Input: part model. Units: mm. Frame: model coordinates. A direction names the side the tool comes from. Round coordinates to 2 decimals unless told otherwise and drop trailing zeros. Order: outer loops, then holes, each group sorted by start corner. A loop starts at its lowest first (then second) coordinate and runs counter-clockwise, first axis right, second up. Notation, with made-up numbers: (25.5, -10) -> (84.5, -10) arc R30 ccw to (84.5, 27) -> close; hole circle Ø4 at (29, -23). An arc over 180 degrees is marked (long way). Use a Markdown table: item, result.
from build123d import *

# Parameters (mm, degrees)
F0_W     = 50
F0_H     = 20
F1_DEPTH = 2
F2_W     = 54
F2_H     = 24
F2_W_2   = 50
F2_H_2   = 20
F3_DEPTH = 8
F4_R     = 0.5


with BuildPart() as f1:
    # F0 (on Top) → F1 (new body)
    with BuildSketch(Plane.XY):
        with Locations((-29.275745, 24.148707)):
            Rectangle(F0_W, F0_H)
    extrude(amount=F1_DEPTH)

    # F2 (on face) → F3 (join)
    with BuildSketch(Plane.XY.offset(2)):
        with Locations((-29.275745, 24.148707)):
            Rectangle(F2_W, F2_H)
        with Locations((-29.275745, 24.148707)):
            Rectangle(F2_W_2, F2_H_2, mode=Mode.SUBTRACT)
    extrude(amount=-F3_DEPTH)

    # F4
    f4_edges = [f1.edges().sort_by_distance(p)[0] for p in [
        (-29.275745, 12.148707, -6),
        (-29.275745, 14.148707, -6),
        (-56.275745, 24.148707, -6),
        (-54.275745, 24.148707, -6),
        (-29.275745, 36.148707, -6),
        (-29.275745, 34.148707, -6),
        (-4.275745, 24.148707, -6),
        (-2.275745, 24.148707, -6),
        (-4.275745, 24.148707, 0),
        (-29.275745, 14.148707, 0),
        (-4.275745, 14.148707, -3),
        (-29.275745, 34.148707, 0),
        (-4.275745, 34.148707, -3),
        (-54.275745, 24.148707, 0),
        (-54.275745, 34.148707, -3),
        (-54.275745, 14.148707, -3),
        (-29.275745, 36.148707, 2),
        (-2.275745, 36.148707, -2),
        (-2.275745, 24.148707, 2),
        (-2.275745, 12.148707, -2),
        (-29.275745, 12.148707, 2),
        (-56.275745, 12.148707, -2),
        (-56.275745, 36.148707, -2),
        (-56.275745, 24.148707, 2),
    ]]
    fillet(f4_edges, radius=F4_R)


solid = f1.part
1) Set-up query: faces 1 (the face through (-56.276, 24, -2)), 2 (the face through (-54.276, 24, -3)). Return all of +Z, -Z, +X, -X, +Y, -Y with unobstructed straight access to the full face (end or side cutting, diameter ignored); none if empty.
Answer key:
| item | result |
|---|---|
| face 1 | +Z, -Z, -X, +Y, -Y |
| face 2 | -Z |
2) Cut plane B-B on y = 23.5. Return loops of the section in (x, z), and give its area (3 significant figures).
Answer key:
| item | result |
|---|---|
| outline | (-56.28, -5.5) arc R0.5 ccw to (-55.78, -6) -> (-54.78, -6) arc R0.5 ccw to (-54.28, -5.5) -> (-54.28, -0.5) arc R0.5 cw to (-53.78, 0) -> (-4.78, 0) arc R0.5 cw to (-4.28, -0.5) -> (-4.28, -5.5) arc R0.5 ccw to (-3.78, -6) -> (-2.78, -6) arc R0.5 ccw to (-2.28, -5.5) -> (-2.28, 1.5) arc R0.5 ccw to (-2.78, 2) -> (-55.78, 2) arc R0.5 ccw to (-56.28, 1.5) -> close |
| area | 132 mm^2 |
3) Cut plane C-C on x = -36. Return loops of the section in (y, z).
Answer key:
| item | result |
|---|---|
| outline | (12.15, -5.5) arc R0.5 ccw to (12.65, -6) -> (13.65, -6) arc R0.5 ccw to (14.15, -5.5) -> (14.15, -0.5) arc R0.5 cw to (14.65, 0) -> (33.65, 0) arc R0.5 cw to (34.15, -0.5) -> (34.15, -5.5) arc R0.5 ccw to (34.65, -6) -> (35.65, -6) arc R0.5 ccw to (36.15, -5.5) -> (36.15, 1.5) arc R0.5 ccw to (35.65, 2) -> (12.65, 2) arc R0.5 ccw to (12.15, 1.5) -> close |
4) Draft query along Y for faces 3 (the face through (-4.276, 24, -3)), 4 (the face through (-30, 34.149, -3)), 5 (the face through (-30, 36.149, -2)), 6 (the face through (-2.276, 24, -2)). Return one class per face: released by +Y, released by -Y, zero draft, split by the parting line, or undercut.
Answer key:
| item | result |
|---|---|
| face 3 | undercut |
| face 4 | undercut |
| face 5 | released by +Y |
| face 6 | zero draft |
5) Cut plane A-A on z = -4. Return loops of the section in (x, y), and give its area (3 significant figures).
Answer key:
| item | result |
|---|---|
| outline | (-56.28, 12.65) arc R0.5 ccw to (-55.78, 12.15) -> (-2.78, 12.15) arc R0.5 ccw to (-2.28, 12.65) -> (-2.28, 35.65) arc R0.5 ccw to (-2.78, 36.15) -> (-55.78, 36.15) arc R0.5 ccw to (-56.28, 35.65) -> close; hole (-54.28, 14.65) arc R0.5 ccw to (-53.78, 14.15) -> (-4.78, 14.15) arc R0.5 ccw to (-4.28, 14.65) -> (-4.28, 33.65) arc R0.5 ccw to (-4.78, 34.15) -> (-53.78, 34.15) arc R0.5 ccw to (-54.28, 33.65) -> close |
| area | 296 mm^2 |
6) Contact query for flat-ended pins moving along their axis: P1, Ø12, axis at x = -42, y = 33.5, coming from the -Z side; P2, Ø3, axis at x = -24.5, y = 28, coming from the -Z side. Output: stop coordinate, or through.
Answer key:
| item | result |
|---|---|
| P1 | stops at z = -6 |
| P2 | stops at z = 0 |
7) Ray query, probe 1 along X at (y, z) = (23, -1); probe 2 along Y at (x, z) = (-14, -5.5); probe 3 along Z at (x, y) = (-31, 17.25). Return the intervals inside material, ascending.
Answer key:
| item | result |
|---|---|
| probe 1 | x = -56.28 to -54.28, -4.28 to -2.28 |
| probe 2 | y = 12.15 to 14.15, 34.15 to 36.15 |
| probe 3 | z = 0 to 2 |
